from build123d import *

# Parameters (mm, degrees)
SKETCH_1_W      = 300
SKETCH_1_H      = 200
EXTRUDE_1_DEPTH = 0.75
SKETCH_2_W      = 297
SKETCH_2_H      = 197
EXTRUDE_2_DEPTH = 0.75


with BuildPart() as part:
    # Эскиз1 → Бобышка-Вытянуть1 (new body)
    with BuildSketch(Plane(origin=(0, 0, 0), x_dir=(0, 0, -1), z_dir=(1, 0, 0))):
        Rectangle(SKETCH_1_W, SKETCH_1_H)
    extrude(amount=-EXTRUDE_1_DEPTH)

    # Эскиз2 → Бобышка-Вытянуть2 (add)
    with BuildSketch(Plane.ZY.offset(0.75)):
        Rectangle(SKETCH_2_W, SKETCH_2_H)
    extrude(amount=EXTRUDE_2_DEPTH)


solid = part.part
The model under review builds one solid part; all positions refer to its coordinate system, in mm. Coordinates: 2 decimals unless noted, no trailing zeros. Write each loop counter-clockwise with the first axis right and the second up, starting at its lowest first coordinate (ties: lowest second). Pieces come first, ordered by that corner, then holes. Notation, with made-up numbers: (74, 37.5) -> (105, 37.5) arc R28 cw to (105, 56.5) -> close; hole circle Ø2 at (33.5, -33.75). An arc over 180 degrees is marked (long way). Answer in a Markdown table with one row per item.
1. Clearance check with a flat-ended pin moving along its axis: pin 1 Ø0.6 at (x, y) = (-1, 4) entering from +Z. State where the tip first meets the part, or that it passes through.
Answers below:
| item | result |
|---|---|
| pin 1 | stops at z = 150 |
2. We need section A-A, the plane x = -1.05. State the section outline as (y, z) points, and give its area (3 significant figures).
Answers below:
| item | result |
|---|---|
| outline | (-98.5, -148.5) -> (98.5, -148.5) -> (98.5, 148.5) -> (-98.5, 148.5) -> close |
| area | 58,500 mm^2 |
3. Wall thickness on probe 1 along Y at (x, z) = (-0.8, 23.5); probe 2 along Z at (x, y) = (-1.1, -90.5): over which ranges is each line inside the solid? List them lowest first. Write a range as [from, to].
Answers below:
| item | result |
|---|---|
| probe 1 | y = [-98.5, 98.5] |
| probe 2 | z = [-148.5, 148.5] |
